from build123d import *

# Parameters (mm, degrees)
EXTRUDE_1_DEPTH = 24
CHAMFER_1_SIZE  = 1


with BuildPart() as part:
    # Эскиз1 → Бобышка-Вытянуть1 (new body)
    with BuildSketch(Plane(origin=(0, 0, 0), x_dir=(0, 0, -1), z_dir=(1, 0, 0))):
        Polygon((0, 5.773502692), (-5, 2.886751346), (-5, -2.886751346), (0, -5.773502692), (5, -2.886751346), (5, 2.886751346), align=None)
    extrude(amount=EXTRUDE_1_DEPTH)

    # Эскиз2 → Вырез-Повернуть1 (revolve, cut)
    with BuildSketch(Plane.XY, mode=Mode.PRIVATE) as cut_revolve_1_sk:
        Polygon((3.196152423, 5.773502692), (8, 3), (24, 3), (24, 5.773502692), align=None)
    revolve(cut_revolve_1_sk.sketch.rotate(Axis((0, 0, 0), (1, 0, 0)), 90), axis=Axis((0, 0, 0), (1, 0, 0)), mode=Mode.SUBTRACT)

    # Фаска1
    chamfer_1_edges = [part.edges().sort_by_distance(p)[0] for p in [
        (24, 0, -3),
    ]]
    chamfer(chamfer_1_edges, length=CHAMFER_1_SIZE)


solid = part.part
The listing builds one solid part. Answer for the finished solid, in the listing's coordinates (mm). A direction names the side the tool comes from. Round coordinates to 2 decimals unless told otherwise and drop trailing zeros. Loops run counter-clockwise (first coordinate to the right, second up) from the corner with the lowest first, then second, coordinate; pieces in that order, holes last. Notation, with made-up numbers: M -39.75,7 L -26.75,7 A20 ccw -26.75,17 Z; hole C 66.5,30 d5. An arc over 180 degrees is marked long. Return JSON: item names as keys, results as strings.
Q1. Find section B-B, the plane x = 1.75. Determine the outline of the cut face in (y, z).
Results list:
{"outline": "M -5.77,0 L -2.89,-5 L 2.89,-5 L 5.77,0 L 2.89,5 L -2.89,5 Z"}
Q2. Each of these flat-tipped pins is pushed along its axis until it touches: pin 1 Ø2 at (y, z) = (-3.5, 2) entering from -X; pin 2 Ø2 at (x, z) = (3, 3.5) entering from +Y; pin 3 Ø1.5 at (x, y) = (18, -4) entering from -Z; pin 4 Ø1 at (x, y) = (10.5, -2) entering from +Z. Where does it stop, or does it pass through?
Results list:
{"pin 1": "stops at x = 0", "pin 2": "stops at y = 4.33", "pin 3": "passes through", "pin 4": "stops at z = 2.6"}
Q3. Find the intervals of material crossed by line 1 along X through (y, z) = (3.5, -0.75); line 2 along Y through (x, z) = (16.75, -0.5); line 3 along Z through (x, y) = (15.5, 1.25), in increasing order. Write a range as from..to.
Results list:
{"line 1": "x = 0..7", "line 2": "y = -2.96..2.96", "line 3": "z = -2.73..2.73"}
Q4. Which of the six approach directions +Z, -Z, +X, -X, +Y, -Y give full straight-line access (tool end or side, diameter ignored) to faces 1 (the face through (2, 0, -5)), 2 (the face through (15.6, -0.9, 2.86))?
Results list:
{"face 1": "-Z, +X, -X, +Y, -Y", "face 2": "+X"}
Q5. Find section A-A, the plane y = 0. Determine the outline of the cut face in (x, z).
Results list:
{"outline": "M 0,-5 L 4.54,-5 L 8,-3 L 23,-3 L 24,-2 L 24,2 L 23,3 L 8,3 L 4.54,5 L 0,5 Z"}
